Work out the finished part from the listing and answer in its coordinate system (mm). A direction names the side the tool comes from. Round coordinates to 2 decimals unless told otherwise and drop trailing zeros. Loops run counter-clockwise (first coordinate to the right, second up) from the corner with the lowest first, then second, coordinate; pieces in that order, holes last. Notation, with made-up numbers: M -27,71 L 26,71 A5 ccw 26,77 Z; hole C 59,31 d8. An arc over 180 degrees is marked long. One line per item, written item: value.
Autodesk Inventor part; units mm, degrees
ref_plane "YZ Plane" through (0, 0, 0) normal (1, 0, 0) x (0, 1, 0)
ref_plane "XZ Plane" through (0, 0, 0) normal (0, 1, 0) x (-1, 0, 0)
ref_plane "XY Plane" through (0, 0, 0) normal (0, 0, 1) x (1, 0, 0)
sketch "Sketch2" plane through (0, 0, 0) normal (0, 1, 0) x (-1, 0, 0)
  line L0 (22.5, -20) -> (-22.5, -20)
  line L1 (-22.5, -20) -> (-22.5, -30.9)
  line L2 (-22.5, -30.9) -> (22.5, -30.9)
  line L3 (22.5, -30.9) -> (22.5, -20)
  line L4 (0, -37.08) -> (0, 6.18) construction
  line L5 (40, 0) -> (-40, 0)
  line L6 (-40, 0) -> (-40, -20)
  line L7 (-40, -20) -> (40, -20)
  line L8 (40, -20) -> (40, 0)
  circle A0 centre (34.25, -10) radius 2.75
  circle A1 centre (-34.25, -10) radius 2.75
  point P0 (0, 0)
  point P1 (0, -20)
  point P2 (-22.5, -20)
  dimension "d0" = 45
  dimension "d1" = 22.5
  dimension "d2" = 10.9
  dimension "d3" = 5.5
  dimension "d4" = 68.5
  dimension "d5" = 34.25
  dimension "d6" = 40
  dimension "d7" = 40
  dimension "d8" = 20
  dimension "d9" = 10
  dimension "d10" = 5.5
  dimension "d11" = 10
extrude "Extrusion1" add sketch "Sketch2" along normal blind 4
sketch "Sketch3" plane through (22.5, 0, -20) normal (1, 0, 0) x (0, 0, -1)
  line L0 (0, 0) -> (10.9, 0) construction
  line L1 (10.9, 0) -> (10.9, 4) construction
  line L2 (0, 4) -> (10.9, 4) construction
  line L3 (0, 0) -> (0, 4) construction
  line L4 (10.9, 4) -> (8.9, 4)
  line L5 (8.9, 4) -> (8.9, 17.75)
  line L6 (9.9, 18.75) -> (10.9, 18.75)
  line L7 (10.9, 15.75) -> (10.9, 4)
  line L8 (10.9, 18.75) -> (23.9, 18.75)
  line L9 (23.9, 18.75) -> (23.9, 16.75)
  line L10 (23.9, 16.75) -> (11.9, 16.75)
  line L11 (8.9, 0) -> (10.9, 0)
  line L12 (10.9, 0) -> (10.9, -5.75)
  line L13 (10.9, -8.75) -> (9.9, -8.75)
  line L14 (8.9, -7.75) -> (8.9, 0)
  line L15 (10.9, -8.75) -> (23.9, -8.75)
  line L16 (23.9, -8.75) -> (23.9, -6.75)
  line L17 (23.9, -6.75) -> (11.9, -6.75)
  arc A0 (11.9, 16.75) -> (10.9, 15.75) centre (11.9, 15.75) ccw
  arc A1 (9.9, 18.75) -> (8.9, 17.75) centre (9.9, 17.75) ccw
  arc A2 (8.9, -7.75) -> (9.9, -8.75) centre (9.9, -7.75) ccw
  arc A3 (10.9, -5.75) -> (11.9, -6.75) centre (11.9, -5.75) ccw
  point P0 (-20, 0)
  dimension "d14" = 6.75
  dimension "d15" = 12.75
  dimension "d16" = 2
  dimension "d17" = 2
  dimension "d18" = 2
  dimension "d19" = 13
  dimension "d20" = 1
  dimension "d21" = 15
extrude "Extrusion2" add sketch "Sketch3" against normal up to surface (45 mm away)
fillet "Fillet1" radius 2 2 edges at (0, 0, -28.9) (0, 4, -28.9)
sketch "Sketch4" plane through (22.5, 18.75, -29.9) normal (0, 1, 0) x (1, 0, 0)
  line L0 (-45, 14) -> (-45, 0) construction
  line L1 (0, 0) -> (-45, 0) construction
  line L2 (0, 14) -> (0, 0) construction
  line L3 (0, 14) -> (-45, 14) construction
  line L4 (-22.5, 26.78) -> (-22.5, -62.68) construction
  point P0 (-22.5, -29.9)
  point P1 (-37.5, 7)
  point P2 (-7.5, 7)
  dimension "d25" = 15
  dimension "d26" = 15
  dimension "d27" = 7
  dimension "d28" = 7
hole "Hole1" at (15, 18.75, -36.9) at (-15, 18.75, -36.9) direction (0, -1, 0) diameter 2.459 depth 27.5
fillet "Fillet2" radius 2 6 edges at (22.5, 2, -20) (40, 2, -20) (40, 2, 0) (-40, 2, 0) (-40, 2, -20) (-22.5, 2, -20)
equation "\"d5\" = 0.5 * d4"
equation "\"d9\" = 0.5 * d8"
properties part number "P047_BoitierCouvercleV4_porteLidar"
1) Find section A-A (z = -10). Give the vertices of the cut face in (x, y), then the cut area to 3 significant figures.
Check values:
outline: M -40,0 L -37,0 L -37,4 L -40,4 Z; M -31.5,0 L 31.5,0 L 31.5,4 L -31.5,4 Z; M 37,0 L 40,0 L 40,4 L 37,4 Z
area: 276 mm2
2) The mould has two halves that part along Y. Classify faces 1 (the face through (-39.43, 2.03, -0.6)), 2 (the face through (0, -8.75, -37)), 3 (the face through (0, 16.75, -38)): +Y half, -Y half, draft (parallel to the pull), parting line (faces both ways), or undercut.
Check values:
face 1: draft
face 2: -Y half
face 3: undercut
3) For faces 4 (the face through (0, 5, -30.9)), 5 (the face through (0, -5, -28.9)), 6 (the face through (23.07, 2.03, -20.6)), determine the directions among +Z, -Z, +X, -X, +Y, -Y from which every point of the face is accessible in a straight line to the end or side of a thin tool.
Check values:
face 4: -Z, +X, -X
face 5: +Z, +X, -X, -Y
face 6: -Z, +X, +Y, -Y
4) Find the intervals of material crossed by probe 1 along X at (y, z) = (-7.9, -36.9); probe 2 along Z at (x, y) = (15, 17.3); probe 3 along Z at (x, y) = (34.25, 1), in increasing order. Write a range as from..to.
Check values:
probe 1: -22.5..-16.23, -13.77..13.77, 16.23..22.5
probe 2: -43.9..-38.13, -35.67..-28.9
probe 3: -20..-12.75, -7.25..0
5) Find section D-D (x = -34.25). Give the vertices of the cut face in (y, z).
Check values:
outline: M 0,-20 L 4,-20 L 4,-12.75 L 0,-12.75 Z; M 0,-7.25 L 4,-7.25 L 4,0 L 0,0 Z
6) Find section C-C (z = -41). Give the vertices of the cut face in (x, y).
Check values:
outline: M -22.5,-8.75 L 22.5,-8.75 L 22.5,-6.75 L -22.5,-6.75 Z; M -22.5,16.75 L 22.5,16.75 L 22.5,18.75 L -22.5,18.75 Z
7) Find section B-B (x = -15). Give the vertices of the cut face in (y, z), then the cut area to 3 significant figures.
Check values:
outline: M -8.75,-43.9 L -6.75,-43.9 L -6.75,-38.13 L -8.75,-38.13 Z; M -8.75,-35.67 L -6.75,-35.67 L -6.75,-31.9 A1 cw -5.75,-30.9 L 15.75,-30.9 A1 cw 16.75,-31.9 L 16.75,-35.67 L 18.75,-35.67 L 18.75,-29.9 A1 ccw 17.75,-28.9 L 6,-28.9 A2 cw 4,-26.9 L 4,0 L 0,0 L 0,-26.9 A2 cw -2,-28.9 L -7.75,-28.9 A1 ccw -8.75,-29.9 Z; M 16.75,-43.9 L 18.75,-43.9 L 18.75,-38.13 L 16.75,-38.13 Z
area: 214 mm2
8) Each of these flat-tipped pins is pushed along its axis until it touches: pin 1 (6.5 mm diameter, centred on x = -4.5, y = -4, fed in from +Z); pin 2 (6.5 mm diameter, centred on x = 34.25, z = -10, fed in from -Y); pin 3 (3 mm diameter, centred on x = 29, y = 2.5, fed in from -Z). Where does it stop, or does it pass through?
Check values:
pin 1: z = -28.46
pin 2: y = 0
pin 3: z = -20
